Check sheet for the modelled part. Datum: model origin and axes. Units: mm. Face numbers are marked on the shaded views. A direction names the side the tool comes from. Coordinates: 2 decimals unless noted, no trailing zeros. Loops run counter-clockwise (first coordinate to the right, second up) from the corner with the lowest first, then second, coordinate; pieces in that order, holes last. Notation, with made-up numbers: M 64.25,-3 L 114.25,-3 A34 ccw 114.25,30 Z; hole C 10,41 d9. An arc over 180 degrees is marked long. Write each question's results on one line, items separated by ' | '. Start each with the question number.
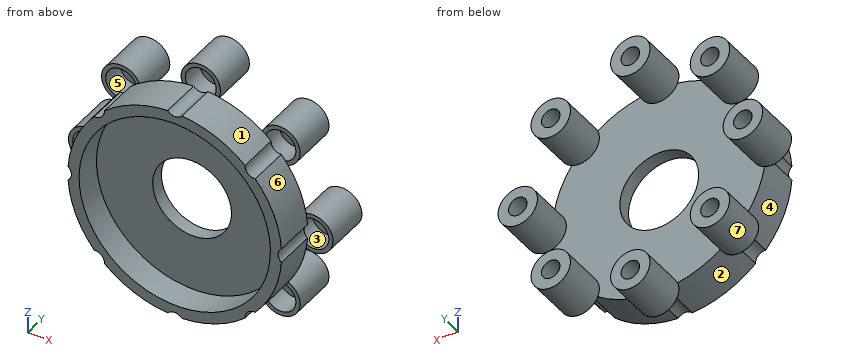
from build123d import *

# Parameters (mm, degrees)
SKETCH3_R               = 8.75
BOSS_EXTRUDE1_DEPTH     = 20
CUT_EXTRUDE1_DEPTH      = 92.362601758
CUT_EXTRUDE1_DEPTH_BACK = 92.362601758
SKETCH4_R               = 4.1
SKETCH5_R               = 6.880501159
CUT_EXTRUDE2_DEPTH      = 10


with BuildPart() as part:
    # Sketch2 → Revolve1 (revolve)
    with BuildSketch(Plane(origin=(0, 0, 0), x_dir=(0, 0, -1), z_dir=(1, 0, 0))):
        Polygon((-47.5, 9), (-47.5, -9), (-42.5, -9), (-42.5, 3), (-17.5, 3), (-17.5, 9), align=None)
    revolve(axis=Axis((0, 40.533381554, 0), (0, -1, 0)))

    # Sketch3 → Boss-Extrude1 (add)
    with BuildSketch(Plane(origin=(0, 9, 0), x_dir=(1, 0, 0), z_dir=(0, 1, 0))):
        with Locations(Location((0, 50, 0), (0, 0, 201.473535129))):
            Circle(SKETCH3_R)
        with Locations(Location((35.355339059, 35.355339059, 0), (0, 0, 156.473535129))):
            Circle(SKETCH3_R)
        with Locations(Location((50, 0, 0), (0, 0, 111.473535129))):
            Circle(SKETCH3_R)
        with Locations(Location((35.355339059, -35.355339059, 0), (0, 0, 66.473535129))):
            Circle(SKETCH3_R)
        with Locations(Location((0, -50, 0), (0, 0, 158.526464871))):
            Circle(SKETCH3_R)
        with Locations(Location((-35.355339059, -35.355339059, 0), (0, 0, 113.526464871))):
            Circle(SKETCH3_R)
        with Locations(Location((-50, 0, 0), (0, 0, 68.526464871))):
            Circle(SKETCH3_R)
        with Locations(Location((-35.355339059, 35.355339059, 0), (0, 0, 23.526464871))):
            Circle(SKETCH3_R)
    extrude(amount=BOSS_EXTRUDE1_DEPTH)

    # Sketch4 → Cut-Extrude1 (cut, two sides: drawn at the far end of the back side and taken through both)
    with BuildSketch(Plane(origin=(0, 29, 0), x_dir=(1, 0, 0), z_dir=(0, 1, 0)).offset(-CUT_EXTRUDE1_DEPTH_BACK)):
        with Locations(Location((0, 50, 0), (0, 0, 270))):
            Circle(SKETCH4_R)
        with Locations(Location((35.355339059, 35.355339059, 0), (0, 0, 270))):
            Circle(SKETCH4_R)
        with Locations(Location((50, 0, 0), (0, 0, 270))):
            Circle(SKETCH4_R)
        with Locations(Location((35.355339059, -35.355339059, 0), (0, 0, 270))):
            Circle(SKETCH4_R)
        with Locations(Location((0, -50, 0), (0, 0, 270))):
            Circle(SKETCH4_R)
        with Locations(Location((-35.355339059, -35.355339059, 0), (0, 0, 270))):
            Circle(SKETCH4_R)
        with Locations(Location((-50, 0, 0), (0, 0, 270))):
            Circle(SKETCH4_R)
        with Locations(Location((-35.355339059, 35.355339059, 0), (0, 0, 270))):
            Circle(SKETCH4_R)
    extrude(amount=CUT_EXTRUDE1_DEPTH + CUT_EXTRUDE1_DEPTH_BACK, mode=Mode.SUBTRACT)

    # Sketch5 → Cut-Extrude2 (cut)
    with BuildSketch(Plane.XZ.offset(-9)):
        with Locations(Location((35.355339059, 35.355339059, 0), (0, 0, 270))):
            Circle(SKETCH5_R)
        with Locations(Location((-35.355339059, 35.355339059, 0), (0, 0, 270))):
            Circle(SKETCH5_R)
        with Locations(Location((-50, 0, 0), (0, 0, 270))):
            Circle(SKETCH5_R)
        with Locations(Location((-35.355339059, -35.355339059, 0), (0, 0, 270))):
            Circle(SKETCH5_R)
        with Locations(Location((0, -50, 0), (0, 0, 270))):
            Circle(SKETCH5_R)
        with Locations(Location((35.355339059, -35.355339059, 0), (0, 0, 270))):
            Circle(SKETCH5_R)
        with Locations(Location((50, 0, 0), (0, 0, 270))):
            Circle(SKETCH5_R)
        with Locations(Location((0, 50, 0), (0, 0, 270))):
            Circle(SKETCH5_R)
    extrude(amount=-CUT_EXTRUDE2_DEPTH, mode=Mode.SUBTRACT)


solid = part.part
Item 1: Tool access check on the marked faces 4, 5, 6 and 7. Record the directions out of +Z, -Z, +X, -X, +Y, -Y that give a thin tool (end or side, any length) a straight path to the whole face; none if there is none.
Item 2: Thickness scan on line 1 (X direction, y = 18.5, z = -35.5); line 2 (X direction, y = 7.25, z = 0); line 3 (X direction, y = 26.5, z = 50). Record the ranges inside material, lowest first.
Item 3: Depth check by flat-ended pin: P1, Ø12, axis at x = 8, y = 0.5, coming from the +Z side; P2, Ø8, axis at x = -25.5, z = -31, coming from the -Y side; P3, Ø12, axis at x = 33, z = -19, coming from the +Y side; P4, Ø10, axis at x = -27.5, y = 10.5, coming from the -Z side. Enter the tip coordinate at first touch or a pass-through.
Item 4: Section check A-A (x = 50). Record the cut outline in (y, z).
Item 5: Section check B-B (z = -50). Record the cut outline in (x, y).
Item 6: Section check C-C (y = 21). State how many separate pieces and enclosed holes the cut face has, plus the area to 3 significant figures.
Item 7: Release check for a two-part mould opening along Z. For the marked faces 1, 2 and 3 record: +Z half, -Z half, draft (parallel to the pull), parting line (faces both ways), or undercut.
Computed values:
1) face 4: -Z, -X, -Y | face 5: none | face 6: +Z, +X, -Y | face 7: +Y
2) line 1: x = -44.1 to -42.23, -28.48 to -26.61, 26.61 to 28.48, 42.23 to 44.1 | line 2: x = -45.9 to -17.5, 17.5 to 45.9 | line 3: x = -8.75 to -4.1, 4.1 to 8.75
3) P1: stops at z = 47.39 | P2: stops at y = -9 | P3: stops at y = 9 | P4: stops at z = -43.63
4) outline: M 9,-8.75 L 29,-8.75 L 29,-4.1 L 19,-4.1 L 19,-6.88 L 9,-6.88 Z; M 9,6.88 L 19,6.88 L 19,4.1 L 29,4.1 L 29,8.75 L 9,8.75 Z
5) outline: M -8.75,9 L -6.88,9 L -6.88,19 L -4.1,19 L -4.1,29 L -8.75,29 Z; M 4.1,19 L 6.88,19 L 6.88,9 L 8.75,9 L 8.75,29 L 4.1,29 Z
6) separate pieces: 8 | enclosed holes: 8 | area: 1,500 mm²
7) face 1: +Z half | face 2: -Z half | face 3: undercut
